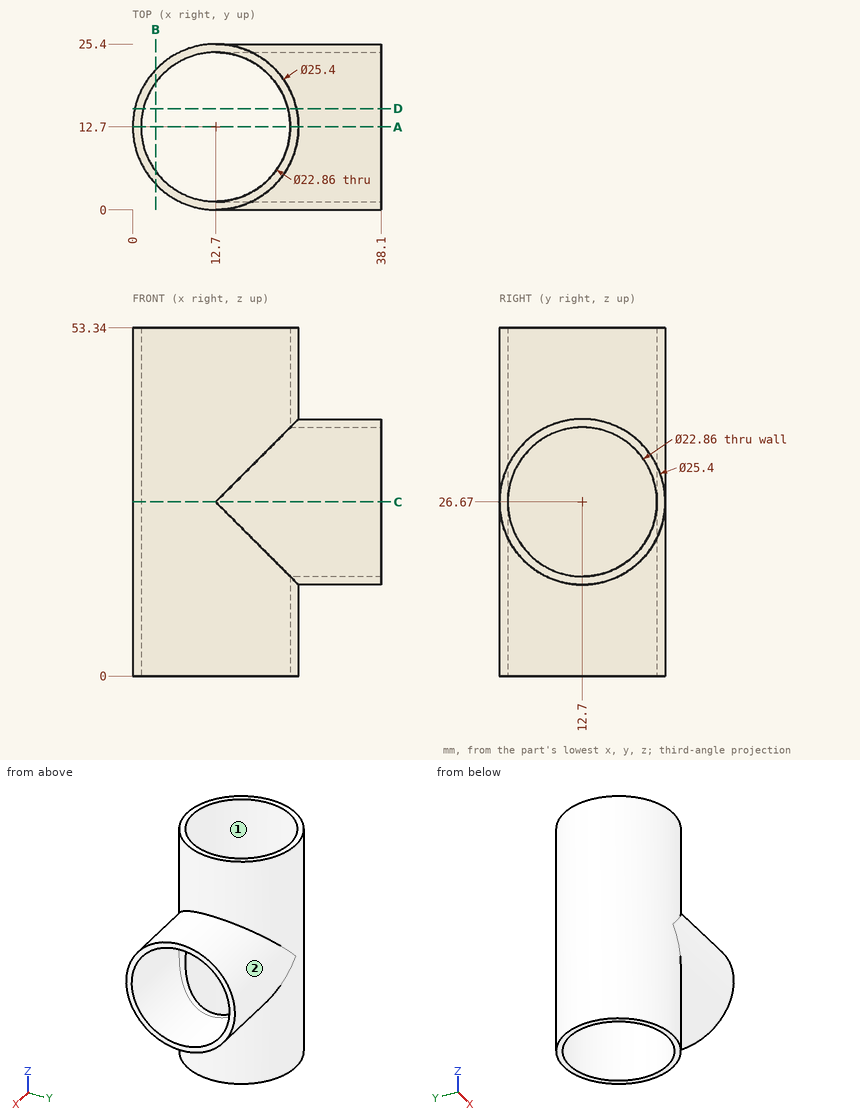
Input: dimensioned drawing with shaded views. Units: mm. Origin: part minimum x, y, z. Round coordinates to 2 decimals unless told otherwise and drop trailing zeros. Loops run counter-clockwise (first coordinate to the right, second up) from the corner with the lowest first, then second, coordinate; pieces in that order, holes last. Notation, with made-up numbers: M -36.5,38.25 L -11.5,38.25 A14 ccw -11.5,64.25 Z; hole C -32.5,16.5 d5. An arc over 180 degrees is marked long. Answer in a Markdown table with one row per item. Add a question column.
1. Section D-D (y = 15.5). Output: boundary loops of the cut face in (x, z), and give its area (3 significant figures).
2. Ray query, probe 1 along Y at (x, z) = (19.25, 26.67); probe 2 along Z at (x, y) = (34, 12.7); probe 3 along Y at (x, z) = (3.5, 46.5) (3 decimals). Return the intervals inside material, ascending.
3. Section A-A (y = 12.7). Output: boundary loops of the cut face in (x, z), and give its area (3 significant figures).
4. Mould query, pull axis Y, two halves, no side actions, for the marked faces 1 and 2. Classes: released by +Y, released by -Y, zero draft, split by the parting line, or undercut.
5. Section C-C (z = 26.67). Output: boundary loops of the cut face in (x, y).
6. Section B-B (x = 3.5). Output: boundary loops of the cut face in (y, z) (3 decimals).
7. Contact query for flat-ended pins moving along their axis: pin 1 (4 mm diameter, centred on x = 5, z = 46, fed in from -Y); pin 2 (8 mm diameter, centred on x = 25, z = 33, fed in from -Y); pin 3 (6 mm diameter, centred on y = 9.5, z = 8.5, fed in from -X). Output: stop coordinate, or through.
Values follow:
| question | item | result |
|---|---|---|
| 1 | outline | M 0.31,0 L 1.62,0 L 1.62,53.34 L 0.31,53.34 Z; M 23.78,0 L 25.09,0 L 25.09,14.28 L 38.1,14.28 L 38.1,15.59 L 23.78,15.59 Z; M 23.78,37.75 L 38.1,37.75 L 38.1,39.06 L 25.09,39.06 L 25.09,53.34 L 23.78,53.34 Z |
| 1 | area | 144 mm^2 |
| 2 | probe 1 | 0 to 1.27, 24.13 to 25.4 |
| 2 | probe 2 | 13.97 to 15.24, 38.1 to 39.37 |
| 2 | probe 3 | 3.945 to 5.917, 19.483 to 21.455 |
| 3 | outline | M 0,0 L 1.27,0 L 1.27,53.34 L 0,53.34 Z; M 24.13,0 L 25.4,0 L 25.4,13.97 L 38.1,13.97 L 38.1,15.24 L 24.13,15.24 Z; M 24.13,38.1 L 38.1,38.1 L 38.1,39.37 L 25.4,39.37 L 25.4,53.34 L 24.13,53.34 Z |
| 3 | area | 139 mm^2 |
| 4 | face 1 | undercut |
| 4 | face 2 | split by the parting line |
| 5 | outline | M 12.7,0 L 38.1,0 L 38.1,1.27 L 12.7,1.27 A11.43 cw 12.7,24.13 L 38.1,24.13 L 38.1,25.4 L 12.7,25.4 A12.7 ccw Z |
| 6 | outline | M 3.945,0 L 5.917,0 L 5.917,53.34 L 3.945,53.34 Z; M 19.483,0 L 21.455,0 L 21.455,53.34 L 19.483,53.34 Z |
| 7 | pin 1 | y = 1.35 |
| 7 | pin 2 | y = 0.22 |
| 7 | pin 3 | x = 0 |
